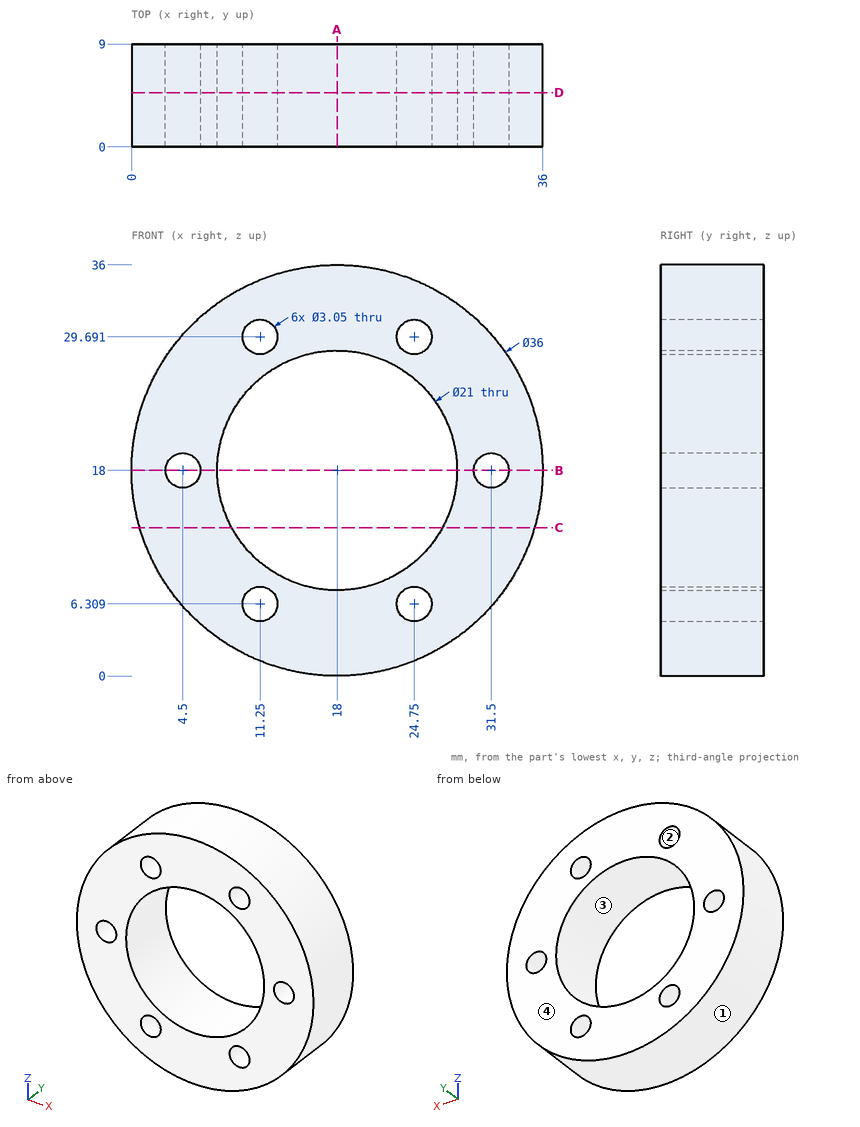
Check sheet for the drawn part. Datum: minimum x, y, z corner. Units: mm. Round coordinates to 2 decimals unless told otherwise and drop trailing zeros. Loops run counter-clockwise (first coordinate to the right, second up) from the corner with the lowest first, then second, coordinate; pieces in that order, holes last. Notation, with made-up numbers: (0.25, 78) - (19.25, 78) arc R4 ccw to (19.25, 85) - close; hole circle Ø2 at (-24, -14). An arc over 180 degrees is marked (long way). Answer as a JSON object with one key per item and string values. Group by question number.
Q1. Sectioned sample at A-A, the plane x = 18. Enter the section's corners in (y, z).
Q2. Sectioned sample at D-D, the plane y = 4.75. Count the separate pieces of the cut face and the enclosed holes in it, plus the area to 3 significant figures.
Q3. Sectioned sample at C-C, the plane z = 13. Enter the section's corners in (x, y), plus the area to 3 significant figures.
Q4. Scan lines: line 1 along Z through (x, y) = (24.75, 3.5) (1 decimal); line 2 along X through (y, z) = (3.75, 29.5); line 3 along X through (y, z) = (5, 17.5). Record each from-to range of solid material in increasing order. Write a range as [from, to].
Q5. Mould release check, pull along X, two halves, no side actions. Record for the marked faces 1, 2, 3 and 4: released by +X, released by -X, zero draft, split by the parting line, or undercut.
Q6. Gauge pin test, flat ends, axial feed: P1, Ø17, axis at x = 18, z = 18, coming from the +Y side; P2, Ø1.5, axis at x = 28, y = 7, coming from the +Z side; P3, Ø4, axis at y = 5, z = 30, coming from the +X side; P4, Ø1, axis at x = 30, y = 1.5, coming from the -Z side. Record the tip position at first contact, or that the pin passes through.
Q7. Sectioned sample at B-B, the plane z = 18. Enter the section's corners in (x, y) (1 decimal).
Solution:
{
 "1": {"outline": "(0, 0) - (9, 0) - (9, 7.5) - (0, 7.5) - close; (0, 28.5) - (9, 28.5) - (9, 36) - (0, 36) - close"},
 "2": {"separate pieces": "1", "enclosed holes": "7", "area": "628 mm²"},
 "3": {"outline": "(0.71, 0) - (8.77, 0) - (8.77, 9) - (0.71, 9) - close; (27.23, 0) - (35.29, 0) - (35.29, 9) - (27.23, 9) - close", "area": "145 mm²"},
 "4": {"line 1": "z = [1.3, 4.8], [7.8, 10], [26, 28.2], [31.2, 34.7]", "line 2": "x = [4.15, 9.74], [12.76, 23.24], [26.26, 31.85]", "line 3": "x = [0.01, 3.06], [5.94, 7.51], [28.49, 30.06], [32.94, 35.99]"},
 "5": {"face 1": "split by the parting line", "face 2": "undercut", "face 3": "undercut", "face 4": "zero draft"},
 "6": {"P1": "passes through", "P2": "stops at z = 33.44", "P3": "stops at x = 32.97", "P4": "stops at z = 4.15"},
 "7": {"outline": "(0, 0) - (3, 0) - (3, 9) - (0, 9) - close; (6, 0) - (7.5, 0) - (7.5, 9) - (6, 9) - close; (28.5, 0) - (30, 0) - (30, 9) - (28.5, 9) - close; (33, 0) - (36, 0) - (36, 9) - (33, 9) - close"}
}
